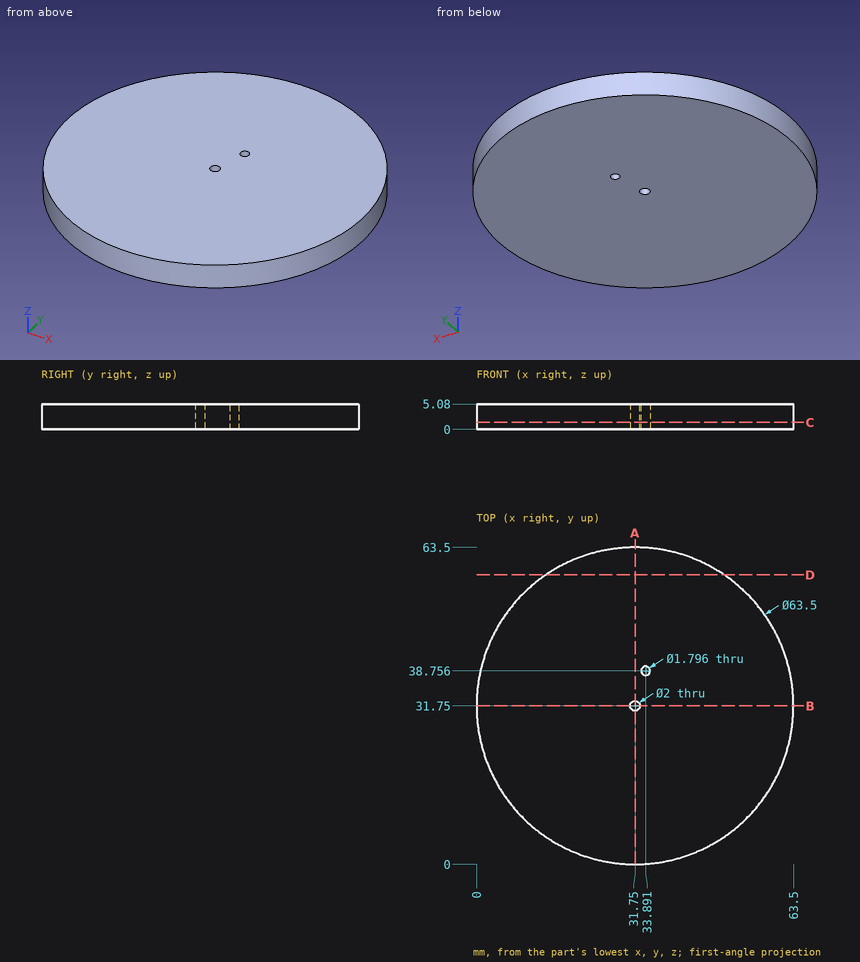
Geometry: see drawing. Coordinates: mm, zero at the bounding-box minimum. Give positions to 0.01 mm unless a question says otherwise; leave off trailing zeros. Order: outer loops, then holes, each group sorted by start corner. A loop starts at its lowest first (then second) coordinate and runs counter-clockwise, first axis right, second up. Notation, with made-up numbers: (75.25, 67.5) - (127.25, 67.5) arc R24 cw to (127.25, 90.5) - close; hole circle Ø2 at (-15, -22.75). An arc over 180 degrees is marked (long way). Use a Markdown table: item, result.
(1) Pin query (flat end, axial travel): pin 1 (1 mm diameter, centred on y = 29.5, z = 4.5, fed in from -X). Return the tip coordinate at first contact, or that it passes through.
Computed values:
| item | result |
|---|---|
| pin 1 | stops at x = 0.05 |
(2) Section query A-A (x = 31.75). Output: boundary loops of the cut face in (y, z).
Computed values:
| item | result |
|---|---|
| outline | (0, 0) - (30.75, 0) - (30.75, 5.08) - (0, 5.08) - close; (32.75, 0) - (63.5, 0) - (63.5, 5.08) - (32.75, 5.08) - close |
(3) Line query: line 1 (Y direction, x = 31, z = 3.3); line 2 (Y direction, x = 43.5, z = 3.85) (1 decimal); line 3 (X direction, y = 51, z = 1.3). Output: solid intervals per line, ascending. Write a range as from..to.
Computed values:
| item | result |
|---|---|
| line 1 | y = 0.01..31.09, 32.41..63.49 |
| line 2 | y = 2.3..61.2 |
| line 3 | x = 6.5..57 |
(4) Section query C-C (z = 1.4). State how many separate pieces and enclosed holes the cut face has, then the cut area to 3 significant figures.
Computed values:
| item | result |
|---|---|
| separate pieces | 1 |
| enclosed holes | 2 |
| area | 3,160 mm2 |
(5) Section query D-D (y = 58). Output: boundary loops of the cut face in (x, z).
Computed values:
| item | result |
|---|---|
| outline | (13.89, 0) - (49.61, 0) - (49.61, 5.08) - (13.89, 5.08) - close |
